For this review, take the finished solid that the model builds, in its own axes (mm). A direction names the side the tool comes from. Give positions to 0.01 mm unless a question says otherwise; leave off trailing zeros. Order: outer loops, then holes, each group sorted by start corner. A loop starts at its lowest first (then second) coordinate and runs counter-clockwise, first axis right, second up.
Item 1: For probe 1 along Z at (x, y) = (1.5, 22); probe 2 along Z at (x, y) = (1.5, 6); probe 3 along Z at (x, y) = (-0.5, 17), list the stretches that pass through material, from the lowest coordinate up.
Item 2: Consider section C-C (z = 57). Give the boundary of the cut face in (x, y), plus the area to 3 significant figures.
Item 3: The part is to be moulded in two halves that separate along Z. For faces 1 (the cylindrical face through (1.276, 10.55, 3.714)), 2 (the flat face through (7.675, 10, 33)), 3 (the flat face through (1, 12, -17.911)), say which applies: released by +Z, released by -Z, zero draft, split by the parting line, or undercut.
Item 4: Machinability: for faces 4 (the cylindrical face through (1.53, 22.61, 64.23)), 5 (the flat face through (1, 25, -8)), which of the approach directions +Z, -Z, +X, -X, +Y, -Y give a long, thin tool a straight path to every point of the face, cutting with its end or side? Answer none if there is none.
Item 5: Consider section B-B (y = 22.5). Give the boundary of the cut face in (x, z).
Item 6: Consider section D-D (x = 2.5). Give the number of separate pieces and of enclosed holes in the cut face, plus the area to 3 significant figures.
Item 7: Consider section A-A (y = 13). Give the boundary of the cut face in (x, z), plus the area to 3 significant figures.
Item 8: For P1, Ø4, axis at x = 0, z = 55.5, coming from the +Y side, flat-tipped, find the tip position at first contact; note if it passes through.
```python
from build123d import *

# Parameters (mm, degrees)
SKETCH1_W                                    = 12.5
SKETCH1_H                                    = 100
BOSS_EXTRUDE1_DEPTH                          = 25
CBORE_FOR_1_4_BINDING_HEAD_MACHINE_S_2_COUNT = 2
CBORE_FOR_1_4_BINDING_HEAD_MACHINE_S_2_PITCH = 50
CUT_EXTRUDE1_REACH                           = 14.5
SKETCH4_R                                    = 4.445


with BuildPart() as part:
    # Sketch1 → Boss-Extrude1 (new body)
    with BuildSketch(Plane(origin=(0, 0, 0), x_dir=(1, 0, 0), z_dir=(0, 1, 0))):
        with Locations((1.425031038, -32.088839839)):
            Rectangle(SKETCH1_W, SKETCH1_H)
    extrude(amount=BOSS_EXTRUDE1_DEPTH)

    # Sketch3 → CBORE for 1/4 Binding Head Machine Screw1 (revolve, cut)
    with BuildSketch(Plane(origin=(1.425031038, 25, 7.088839839), x_dir=(0, 0, 1), z_dir=(1, 0, 0))):
        Polygon((0, 0), (0, 25), (3.3782, 25), (3.3782, 4.191), (7.14375, 4.191), (7.14375, 0.635), (7.77875, 0), align=None)
    cbore_for_1_4_binding_head_machine_screw = revolve(axis=Axis((1.425031038, 31.35, 7.088839839), (0, -1, 0)), mode=Mode.SUBTRACT)

    # CBORE for 1_4 Binding Head Machine S 2: CBORE for 1/4 Binding Head Machine Screw1 ×2
    with Locations(*[(0, 0, i * CBORE_FOR_1_4_BINDING_HEAD_MACHINE_S_2_PITCH) for i in range(1, CBORE_FOR_1_4_BINDING_HEAD_MACHINE_S_2_COUNT)]):
        add(cbore_for_1_4_binding_head_machine_screw, mode=Mode.SUBTRACT)

    # Sketch4 → Cut-Extrude1 (cut, up to next)
    with BuildSketch(Plane.ZY.offset(4.824968962), mode=Mode.PRIVATE) as cut_extrude1_sk1:
        with Locations((32.088839839, 16)):
            Circle(SKETCH4_R)
    cut_extrude1_tool1 = extrude(cut_extrude1_sk1.sketch, amount=-CUT_EXTRUDE1_REACH, mode=Mode.PRIVATE) & part.part
    add(cut_extrude1_tool1.solids().sort_by_distance((-4.824969, 16, 32.08884))[0], mode=Mode.SUBTRACT)


solid = part.part
```
Resolved:
1. probe 1: z = -17.91 to -0.05, 14.23 to 49.95, 64.23 to 82.09
1. probe 2: z = -17.91 to 3.71, 10.47 to 53.71, 60.47 to 82.09
1. probe 3: z = -17.91 to 4.31, 9.86 to 27.76, 36.42 to 54.31, 59.86 to 82.09
2. outline: (-4.82, 0) - (-1.95, 0) - (-1.95, 20.81) - (-4.82, 20.81) - close; (4.8, 0) - (7.68, 0) - (7.68, 20.81) - (4.8, 20.81) - close
2. area: 120 mm2
3. face 1: undercut
3. face 2: zero draft
3. face 3: released by -Z
4. face 4: +Y
4. face 5: +Z, -Z, +X, -X, +Y
5. outline: (-4.82, -17.91) - (7.68, -17.91) - (7.68, 3.63) arc R7.14 cw to (-4.82, 3.63) - close; (-4.82, 10.55) arc R7.14 cw to (7.68, 10.55) - (7.68, 53.63) arc R7.14 cw to (-4.82, 53.63) - close; (-4.82, 60.55) arc R7.14 cw to (7.68, 60.55) - (7.68, 82.09) - (-4.82, 82.09) - close
6. separate pieces: 3
6. enclosed holes: 1
6. area: 2,050 mm2
7. outline: (-4.82, -17.91) - (7.68, -17.91) - (7.68, 28.81) - (-4.82, 28.81) - close; (-4.82, 35.37) - (7.68, 35.37) - (7.68, 82.09) - (-4.82, 82.09) - close; hole circle Ø6.76 at (1.43, 7.09); hole circle Ø6.76 at (1.43, 57.09)
7. area: 1,100 mm2
8. P1: stops at y = 20.81
